Geometry check sheet. Reference: the model listing, model coordinates, mm. Round coordinates to 2 decimals unless told otherwise and drop trailing zeros. Loops run counter-clockwise (first coordinate to the right, second up) from the corner with the lowest first, then second, coordinate; pieces in that order, holes last. Notation, with made-up numbers: (55, -39) -> (60, -39) arc R14 ccw to (60, -32) -> close; hole circle Ø11 at (85, 11). An arc over 180 degrees is marked (long way). Use a Markdown table: item, result. Add a question column.
Q1. Sectioned sample at C-C, the plane x = -13. Enter the section's corners in (y, z).
Q2. Sectioned sample at B-B, the plane z = 11.5. Enter the section's corners in (x, y).
Q3. Material ranges on L1, parallel to X at y = -914, z = 1.5; L2, parallel to X at y = -433, z = 4; L3, parallel to Z at x = -12, y = -460, recorded low to high.
Q4. Gauge pin test, flat ends, axial feed: P1, Ø1.5, axis at y = -624, z = -13, coming from the -X side; P2, Ø1.5, axis at x = -0.5, z = 1.5, coming from the -Y side; P3, Ø6, axis at y = -205, z = -15, coming from the +X side. Record the tip position at first contact, or that the pin passes through.
```python
from build123d import *

# Parameters (mm, degrees)
F0_W     = 42
F0_H     = 42
F1_DEPTH = 1000
F3_DEPTH = 100
F4_R     = 20.99999


# Not quite as in the source:
# - a fillet or chamfer is up to 0.001 mm smaller than in the source, because OpenCascade refuses the exact size


with BuildPart() as f1:
    # F0 (on Front) → F1 (new body)
    with BuildSketch(Plane.XZ):
        Rectangle(F0_W, F0_H)
    extrude(amount=F1_DEPTH)

    # F2 (on face) → F3 (cut)
    with BuildSketch(Plane.YZ.offset(21)):
        Polygon((-958, -21), (-1000, 21), (-1000, -21), align=None)
    extrude(amount=-F3_DEPTH, mode=Mode.SUBTRACT)

    # F4 (radius 21 in the source; OpenCascade refuses exactly that, so slightly less here)
    f4_edges = [f1.edges().sort_by_distance(p)[0] for p in [
        (21, -500, 21),
        (21, -479, -21),
        (-21, -479, -21),
        (-21, -500, 21),
    ]]
    fillet(f4_edges, radius=F4_R)


solid = f1.part
```
Values:
| question | item | result |
|---|---|---|
| 1 | outline | (-995.49, 16.49) -> (-962.51, -16.49) -> (0, -16.49) -> (0, 16.49) -> close |
| 2 | outline | (-17.57, -990.5) -> (17.57, -990.5) -> (17.57, 0) -> (-17.57, 0) -> close |
| 3 | L1 | -20.95 to 20.95 |
| 3 | L2 | -20.62 to 20.62 |
| 3 | L3 | -17.23 to 17.23 |
| 4 | P1 | x = -17.06 |
| 4 | P2 | y = -981.25 |
| 4 | P3 | x = 17.23 |
